```python
from build123d import *

# Parameters (mm, degrees)
SKETCH1_R           = 4
BOSS_EXTRUDE1_DEPTH = 21
SKETCH3_W           = 15
SKETCH3_H           = 3
BOSS_EXTRUDE2_DEPTH = 15
SKETCH4_R           = 3
CUT_EXTRUDE1_DEPTH  = 1
SKETCH5_R           = 1.5
CUT_EXTRUDE2_DEPTH  = 4
FILLET1_R           = 3
CUT_EXTRUDE3_START  = -27
SKETCH7_R           = 4
CUT_EXTRUDE3_DEPTH  = 27
SKETCH8_R           = 1.5
CUT_EXTRUDE4_DEPTH  = 14
CUT_EXTRUDE5_DEPTH  = 2.5
SKETCH10_R          = 5
CUT_EXTRUDE6_DEPTH  = 7.5


with BuildPart() as part:
    # Sketch1 → Boss-Extrude1 (new body)
    with BuildSketch(Plane.XY):
        with BuildLine():
            ThreePointArc((6.92820323, -4), (0, 8), (-6.92820323, -4))
            Line((-6.92820323, -4), (-7, -4))
            Line((-7, -4), (-7, -8))
            Line((-7, -8), (8, -8))
            Line((8, -8), (8, -4))
            Line((8, -4), (6.92820323, -4))
        make_face()
        with Locations(Location((0, 0, 0), (0, 0, 180))):
            Circle(SKETCH1_R, mode=Mode.SUBTRACT)
    extrude(amount=BOSS_EXTRUDE1_DEPTH)

    # Sketch3 → Boss-Extrude2 (add)
    with BuildSketch(Plane.XZ.offset(8)):
        with Locations((0.5, 19.5)):
            Rectangle(SKETCH3_W, SKETCH3_H)
        with Locations((0.5, 1.5)):
            Rectangle(SKETCH3_W, SKETCH3_H)
    extrude(amount=BOSS_EXTRUDE2_DEPTH)

    # Sketch4 → Cut-Extrude1 (cut)
    with BuildSketch(Plane.XY.offset(21)):
        with Locations((0.5, -15.5)):
            Circle(SKETCH4_R)
    cut_extrude1 = extrude(amount=-CUT_EXTRUDE1_DEPTH, mode=Mode.SUBTRACT)

    # Sketch5 → Cut-Extrude2 (cut, symmetric)
    with BuildSketch(Plane.XY.offset(20)):
        with Locations((0.5, -15.5)):
            Circle(SKETCH5_R)
        with BuildLine():
            Line((2, -18.098076211), (2, -15.5))
            ThreePointArc((2, -15.5), (0.5, -17), (-1, -15.5))
            Line((-1, -15.5), (-1, -18.098076211))
            ThreePointArc((-1, -18.098076211), (0.5, -18.5), (2, -18.098076211))
        make_face()
        with BuildLine():
            Line((2, -23), (2, -18.098076211))
            ThreePointArc((2, -18.098076211), (0.5, -18.5), (-1, -18.098076211))
            Line((-1, -18.098076211), (-1, -23))
            Line((-1, -23), (2, -23))
        make_face()
    cut_extrude2 = extrude(amount=CUT_EXTRUDE2_DEPTH, both=True, mode=Mode.SUBTRACT)

    # Mirror1: Cut-Extrude1, Cut-Extrude2 across plane
    add(cut_extrude1.mirror(Plane.XY.offset(10.5)), mode=Mode.SUBTRACT)
    add(cut_extrude2.mirror(Plane.XY.offset(10.5)), mode=Mode.SUBTRACT)

    # Fillet1
    fillet1_edges = [part.edges().sort_by_distance(p)[0] for p in [
        (8, -23, 19.5),
        (-7, -23, 19.5),
        (8, -23, 1.5),
        (-7, -23, 1.5),
    ]]
    fillet(fillet1_edges, radius=FILLET1_R)

    # Sketch6 → Revolve1 (revolve)
    with BuildSketch(Plane(origin=(0, 0, 0), x_dir=(1, 0, 0), z_dir=(0, 1, 0))):
        Polygon((-9.899494937, -14.899494937), (-6.363961031, -18.435028843), (0, -12.071067812), (-3.535533906, -8.535533906), align=None)
    revolve(axis=Axis((0, 0, 5), (-0.7071067811865487, 0, 0.7071067811865465)))

    # Sketch7 → Cut-Extrude3 (cut)
    with BuildSketch(Plane.XY.offset(21).offset(CUT_EXTRUDE3_START)):
        with Locations(Location((0, 0, 0), (0, 0, 180))):
            Circle(SKETCH7_R)
    extrude(amount=CUT_EXTRUDE3_DEPTH, mode=Mode.SUBTRACT)

    # Sketch8 → Cut-Extrude4 (cut)
    with BuildSketch(Plane(origin=(-12.399494937, 0, 12.399494937), x_dir=(0.7071067811865464, 0, 0.7071067811865487), z_dir=(-0.7071067811865487, 0, 0.7071067811865464))):
        with Locations((3.535533906, 0)):
            Circle(SKETCH8_R)
    extrude(amount=-CUT_EXTRUDE4_DEPTH, mode=Mode.SUBTRACT)

    # Sketch9 → Cut-Extrude5 (cut)
    with BuildSketch(Plane(origin=(-10.278174593, 0, 10.278174593), x_dir=(0.7071067811865464, 0, 0.7071067811865487), z_dir=(-0.7071067811865487, 0, 0.7071067811865464))):
        Polygon((1.918953152, -2.8), (5.15211466, -2.8), (6.768695413, 0), (5.15211466, 2.8), (1.918953152, 2.8), (0.302372398, 0), align=None)
        Polygon((-2.926090212, -2.8), (-2.926090212, 2.8), (1.918953152, 2.8), (0.302372398, 0), (1.918953152, -2.8), align=None)
    extrude(amount=-CUT_EXTRUDE5_DEPTH, mode=Mode.SUBTRACT)

    # Sketch10 → Cut-Extrude6 (cut)
    with BuildSketch(Plane(origin=(-12.399494937, 0, 12.399494937), x_dir=(0.7071067811865464, 0, 0.7071067811865487), z_dir=(-0.7071067811865487, 0, 0.7071067811865464))):
        with Locations((3.535533906, 0)):
            Circle(SKETCH10_R)
    extrude(amount=CUT_EXTRUDE6_DEPTH, mode=Mode.SUBTRACT)


solid = part.part
```
Part model, mm, in its own coordinate system. A direction names the side the tool comes from. Coordinates: 2 decimals unless noted, no trailing zeros. Loops run counter-clockwise (first coordinate to the right, second up) from the corner with the lowest first, then second, coordinate; pieces in that order, holes last. Notation, with made-up numbers: (32, -34) - (37, -34) arc R24 ccw to (37, -20) - close; hole circle Ø10 at (19.5, 45). An arc over 180 degrees is marked (long way). Write item = value, one per line. Start each with the question number.
Item 1: Cut at D-D, the plane y = -16. Give the cut face in (x, z), and give its area (3 significant figures).
Item 2: Mould opens along X. For faces 5 (the flat face through (-9.064, 1.181, 15.735)), 6 (the flat face through (3, -23, 20)), 7 (the cylindrical face through (0.5, -14, 19)) say: released by +X, released by -X, zero draft, split by the parting line, or undercut.
Item 3: Wall check: L1, parallel to Z at x = 4.75, y = -13; L2, parallel to X at y = -1, z = 13; L3, parallel to Z at x = -7.5, y = 0. Give the ranges that are in metal, low to high. Write a range as from..to.
Item 4: Cut at B-B, the plane x = 0.5. Give the cut face in (y, z), and give its area (3 significant figures).
Item 5: Cut at C-C, the plane z = 4. Give the cut face in (x, y).
Item 6: Cut at A-A, the plane y = -9. Give the cut face in (x, z), and give its area (3 significant figures).
Item 7: Flat gauge pins, fed straight in: pin 1 Ø4 at (x, y) = (-5, 5) entering from -Z; pin 2 Ø5 at (x, y) = (0.5, -15.5) entering from -Z; pin 3 Ø10 at (x, z) = (-3, 10) entering from -Y; pin 4 Ø8 at (y, z) = (-13.5, 5.5) entering from -X. Where does each tip first touch, or does it go through?
Item 8: 3-axis set-ups, long thin cutter, end or side, ignore diameter. For faces 1 (the flat face through (-7.41, 0.04, 9.61)), 2 (the cylindrical face through (0.6, -12.5, 20.5)), 3 (the cylindrical face through (-6.14, -22.1, 19.52)), 4 (the flat face through (-1, -19, 20)): which of +Z, -Z, +X, -X, +Y, -Y reach the whole face in a straight line?
The answers:
q1.outline = (-7, 0) - (-2.46, 0) - (-2.46, 1) - (-1, 1) - (-1, 3) - (-7, 3) - close; (-7, 18) - (-1, 18) - (-1, 20) - (-2.46, 20) - (-2.46, 21) - (-7, 21) - close; (2, 1) - (3.46, 1) - (3.46, 0) - (8, 0) - (8, 3) - (2, 3) - close; (2, 18) - (8, 18) - (8, 21) - (3.46, 21) - (3.46, 20) - (2, 20) - close
q1.area = 66.2 mm2
q2.face_5 = released by -X
q2.face_6 = zero draft
q2.face_7 = undercut
q3.L1 = 0..3, 18..21
q3.L2 = -11.8..-9.58, -4.24..-3.87, 3.87..7.94
q3.L3 = 0..9.52, 14.62..17.3, 19.57..21
q4.outline = (-14, 1) - (-12.5, 1) - (-12.5, 0) - (-3.97, 0) - (-3.97, 21) - (-12.5, 21) - (-12.5, 20) - (-14, 20) - (-14, 18) - (-8, 18) - (-8, 3) - (-14, 3) - close; (3.97, 0) - (7.98, 0) - (7.98, 21) - (3.97, 21) - close
q4.area = 202 mm2
q5.outline = (-7, -8) - (8, -8) - (8, -4) - (6.93, -4) arc R8 ccw (long way) to (-6.93, -4) - (-7, -4) - close; hole circle Ø8 at (0, 0)
q6.outline = (-7, 0) - (8, 0) - (8, 3) - (-7, 3) - close; (-7, 18) - (8, 18) - (8, 21) - (-7, 21) - close
q6.area = 90.0 mm2
q7.pin_1 = 0
q7.pin_2 = 1
q7.pin_3 = -8
q7.pin_4 = -7
q8.face_1 = none
q8.face_2 = +Z
q8.face_3 = +Z, -Z, -X, -Y
q8.face_4 = +Z, -Z, -Y
